from build123d import *

# Parameters (mm, degrees)
CYLINDER_R       = 12
CYLINDER_DEPTH   = 300
EXTRUDE003_DEPTH = 80
SKETCH009_R      = 14
EXTRUDE002_DEPTH = 25


with BuildPart() as cylinder:
    # Cylinder → Cylinder (new body)
    with BuildSketch(Plane.ZY.offset(80)):
        Circle(CYLINDER_R)
    extrude(amount=CYLINDER_DEPTH)


with BuildPart() as extrude003:
    # Sketch010 (on Face2 of Extrude002) → Extrude003 (new body)
    with BuildSketch(Plane.XY.offset(30)):
        with BuildLine():
            Line((30, 11.5), (-26, 11.5))
            Line((-26, 11.5), (-26, 14.999992))
            ThreePointArc((-26, 14.999992), (-26.29289, 15.707104), (-27, 16))
            Line((-27, 16), (-33, 16))
            ThreePointArc((-33, 16), (-33.707107, 15.707107), (-34, 15))
            Line((-34, 15), (-34, -15))
            ThreePointArc((-34, -15), (-33.707107, -15.707107), (-33, -16))
            Line((-33, -16), (-27, -16))
            ThreePointArc((-27, -16), (-26.292893, -15.707107), (-26, -15))
            Line((-26, -15), (-26, -11.5))
            Line((-26, -11.5), (30, -11.5))
            Line((30, -11.5), (30, 11.5))
        make_face()
    extrude(amount=-EXTRUDE003_DEPTH)


with BuildPart() as obj1:
    # Sketch009 → Extrude002 (new body, symmetric)
    with BuildSketch(Plane.XZ):
        with BuildLine():
            ThreePointArc((0, -30), (30, 0), (0, 30))
            Line((0, 30), (-80, 30))
            Line((-80, 30), (-80, -30))
            Line((-80, -30), (0, -30))
        make_face()
        Circle(SKETCH009_R, mode=Mode.SUBTRACT)
    extrude(amount=EXTRUDE002_DEPTH, both=True)

    # Cut003: cut Extrude003
    add(extrude003.part, mode=Mode.SUBTRACT)

    # Fusion: union Cylinder
    add(cylinder.part)


solid = obj1.part
Geometry check sheet. Reference: the model listing, model coordinates, mm. A direction names the side the tool comes from. Coordinates: 2 decimals unless noted, no trailing zeros. Order: outer loops, then holes, each group sorted by start corner. A loop starts at its lowest first (then second) coordinate and runs counter-clockwise, first axis right, second up. Notation, with made-up numbers: (-17, -4) - (20, -4) arc R21 ccw to (20, 1) - close; hole circle Ø1 at (-27.5, 33.25). An arc over 180 degrees is marked (long way). Answer in a Markdown table with one row per item. Add a question column.
1) Gauge pin test, flat ends, axial feed: P1, Ø10, axis at y = 8.5, z = 2.5, coming from the +X side; P2, Ø5, axis at x = -276.5, y = 11.5, coming from the +Z side; P3, Ø17, axis at x = 0, z = 0, coming from the -Y side; P4, Ø3, axis at x = -193, y = -7.5, coming from the -Z side. Record the tip position at first contact, or that the pin passes through.
2) Cross-section at A-A, the plane y = 20. Record the cut outline in (x, z), then the cut area to 3 significant figures.
3) Cross-section at C-C, the plane y = 0. Record the cut outline in (x, z).
4) Material ranges on line 1 along X through (y, z) = (-18, 0); line 2 along X through (y, z) = (15, 0); line 3 along Y through (x, z) = (-24, 24), recorded low to high. Write a range as [from, to].
5) Cross-section at B-B, the plane z = 0. Record the cut outline in (x, y), then the cut area to 3 significant figures.
6) Cross-section at D-D, the plane z = 18. Record the cut outline in (x, y), then the cut area to 3 significant figures.
7) Set-up check for faces 5 (the cylindrical face through (-227.9, 0.53, -11.99)), 6 (the flat face through (-4, 11.5, 14)), 7 (the cylindrical face through (12.932, -18.156, -5.362)): record each of +Z, -Z, +X, -X, +Y, -Y from which the full face is reachable in a straight line by a thin tool's end or side.
8) Release check for a two-part mould opening along Y. For faces 1 (the flat face through (-38, 25, 0)), 2 (the flat face through (-38, -25, 0)), 3 (the flat face through (-34, 0, 0)), 4 (the cylindrical face through (29.993, 18.156, -0.66)) record: +Y half, -Y half, draft (parallel to the pull), parting line (faces both ways), or undercut.
Check result:
| question | item | result |
|---|---|---|
| 1 | P1 | stops at x = 30 |
| 1 | P2 | stops at z = 7.94 |
| 1 | P3 | passes through |
| 1 | P4 | stops at z = -10.39 |
| 2 | outline | (-80, -30) - (0, -30) arc R30 ccw to (0, 30) - (-80, 30) - close; hole circle Ø28 at (0, 0) |
| 2 | area | 5,600 mm² |
| 3 | outline | (-380, -12) - (-80, -12) - (-80, -30) - (-34, -30) - (-34, 30) - (-80, 30) - (-80, 12) - (-380, 12) - close |
| 4 | line 1 | x = [-80, -14], [14, 30] |
| 4 | line 2 | x = [-80, -34], [-26, -14], [14, 30] |
| 4 | line 3 | y = [-25, -11.5], [11.5, 25] |
| 5 | outline | (-380, -12) - (-80, -12) - (-80, -25) - (-14, -25) - (-14, -11.5) - (-26, -11.5) - (-26, -15) arc R1 cw to (-27, -16) - (-33, -16) arc R1 cw to (-34, -15) - (-34, 15) arc R1 cw to (-33, 16) - (-27, 16) arc R1 cw to (-26, 15) - (-26, 11.5) - (-14, 11.5) - (-14, 25) - (-80, 25) - (-80, 12) - (-380, 12) - close; (14, -25) - (30, -25) - (30, -11.5) - (14, -11.5) - close; (14, 11.5) - (30, 11.5) - (30, 25) - (14, 25) - close |
| 5 | area | 10,400 mm² |
| 6 | outline | (-80, -25) - (24, -25) - (24, -11.5) - (-26, -11.5) - (-26, -15) arc R1 cw to (-27, -16) - (-33, -16) arc R1 cw to (-34, -15) - (-34, 15) arc R1 cw to (-33, 16) - (-27, 16) arc R1 cw to (-26, 15) - (-26, 11.5) - (24, 11.5) - (24, 25) - (-80, 25) - close |
| 6 | area | 3,790 mm² |
| 7 | face 5 | -X |
| 7 | face 6 | +Z, -Z, +X |
| 7 | face 7 | +Y, -Y |
| 8 | face 1 | +Y half |
| 8 | face 2 | -Y half |
| 8 | face 3 | undercut |
| 8 | face 4 | draft |
